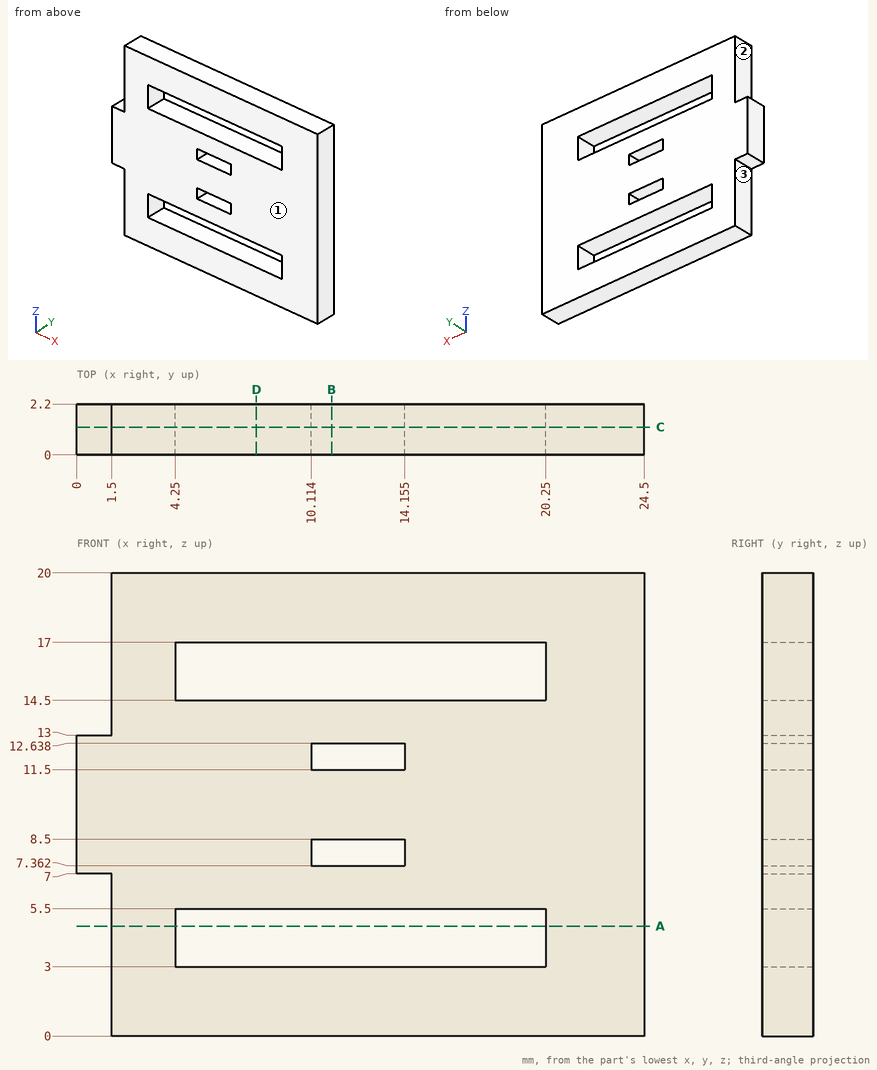
Job drawing, mm, ordinate dimensions from the low corner. One solid piece. A direction names the side the tool comes from. Coordinates: 2 decimals unless noted, no trailing zeros. Write each loop counter-clockwise with the first axis right and the second up, starting at its lowest first coordinate (ties: lowest second). Pieces come first, ordered by that corner, then holes. Notation, with made-up numbers: M 73.25,23.25 L 121.25,23.25 A14 cw 121.25,45.25 Z; hole C 40,36.25 d3. An arc over 180 degrees is marked long. Answer as a JSON object with one key per item and string values. Group by question number.
1) Saw through at A-A (z = 4.75). Write the cut outline in (x, y), plus the area to 3 significant figures.
2) Pin check, flat tips, straight feed: pin 1 Ø0.8 at (x, y) = (1, 0.5) entering from -Z; pin 2 Ø0.7 at (y, z) = (1, 4.5) entering from -X. Stop position of each tip, or through.
3) Saw through at B-B (x = 11). Write the cut outline in (y, z).
4) Wall check: line 1 (Z direction, x = 13, y = 1.8); line 2 (Z direction, x = 9.5, y = 0.3); line 3 (X direction, y = 1.65, z = 5). Give the ranges that are in metal, low to high. Write a range as from..to.
5) Saw through at C-C (y = 1.2). Give the number of separate pieces and of enclosed holes in the cut face, plus the area to 3 significant figures.
6) Saw through at D-D (x = 7.75). Write the cut outline in (y, z), plus the area to 3 significant figures.
7) Tool access for the marked faces 1, 2 and 3: list every direction of +Z, -Z, +X, -X, +Y, -Y with a clear straight run to the whole face (end or side of a thin tool).
Values follow:
{
 "1": {"outline": "M 1.5,0 L 4.25,0 L 4.25,2.2 L 1.5,2.2 Z; M 20.25,0 L 24.5,0 L 24.5,2.2 L 20.25,2.2 Z", "area": "15.4 mm2"},
 "2": {"pin 1": "stops at z = 7", "pin 2": "stops at x = 1.5"},
 "3": {"outline": "M 0,0 L 2.2,0 L 2.2,3 L 0,3 Z; M 0,5.5 L 2.2,5.5 L 2.2,7.36 L 0,7.36 Z; M 0,8.5 L 2.2,8.5 L 2.2,11.5 L 0,11.5 Z; M 0,12.64 L 2.2,12.64 L 2.2,14.5 L 0,14.5 Z; M 0,17 L 2.2,17 L 2.2,20 L 0,20 Z"},
 "4": {"line 1": "z = 0..3, 5.5..7.36, 8.5..11.5, 12.64..14.5, 17..20", "line 2": "z = 0..3, 5.5..14.5, 17..20", "line 3": "x = 1.5..4.25, 20.25..24.5"},
 "5": {"separate pieces": "1", "enclosed holes": "4", "area": "380 mm2"},
 "6": {"outline": "M 0,0 L 2.2,0 L 2.2,3 L 0,3 Z; M 0,5.5 L 2.2,5.5 L 2.2,14.5 L 0,14.5 Z; M 0,17 L 2.2,17 L 2.2,20 L 0,20 Z", "area": "33.0 mm2"},
 "7": {"face 1": "+Z, -Z, +X, -X, -Y", "face 2": "+Z, -X, +Y, -Y", "face 3": "-Z, -X, +Y, -Y"}
}
